Verification items for the finished model (mm, model axes). Face numbers are marked on the shaded views. A direction names the side the tool comes from. Coordinates: 2 decimals unless noted, no trailing zeros. Order: outer loops, then holes, each group sorted by start corner. A loop starts at its lowest first (then second) coordinate and runs counter-clockwise, first axis right, second up. Notation, with made-up numbers: M 57.25,-24 L 107.25,-24 A20 ccw 107.25,-15 Z; hole C -11.5,4 d9. An arc over 180 degrees is marked long. Write item = value, one per line.
```python
from build123d import *

# Parameters (mm, degrees)
BASE_FLANGE1_DEPTH = 2
EDGE_FLANGE1_DEPTH = 1017


# Sheet-metal steps are written as plain solids
with BuildPart() as part:
    # Sketch1 → Base-Flange1 (new body)
    with BuildSketch(Plane.XY):
        Polygon((960.416808149, 91.455857385), (985.416808149, 91.455857385), (985.416808149, 141.455857385), (-231.583191851, 141.455857385), (-231.583191851, 91.455857385), (-206.583191851, 91.455857385), (-206.583191851, -158.544142615), (960.416808149, -158.544142615), align=None)
    extrude(amount=-BASE_FLANGE1_DEPTH)

    # Edge-Flange1 section (across the edge) → Edge-Flange1 (add)
    with BuildSketch(Plane(origin=(-131.583191851, 142.192457385, -2), x_dir=(0, -1, 0), z_dir=(1, 0, 0))):
        with BuildLine():
            Line((-2, 0.7366), (-2, 13))
            Line((-2, 13), (0, 13))
            Line((0, 13), (0, 0.7366))
            ThreePointArc((0, 0.7366), (0.215745145, 0.215745145), (0.7366, 0))
            Line((0.7366, 0), (0.7366, -2))
            ThreePointArc((0.7366, -2), (-1.198468417, -1.198468417), (-2, 0.7366))
        make_face()
    extrude(amount=EDGE_FLANGE1_DEPTH)


solid = part.part
```
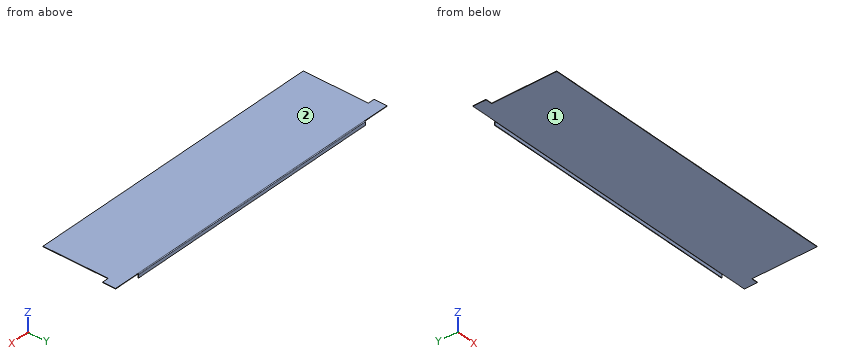
Item 1: Tool access check on the marked faces 1 and 2. Record the directions out of +Z, -Z, +X, -X, +Y, -Y that give a thin tool (end or side, any length) a straight path to the whole face; none if there is none.
Report:
face_1 = -Z, +X, -X, -Y
face_2 = +Z, +X, -X, +Y, -Y
Item 2: Gauge pin test, flat ends, axial feed: pin 1 (0.6 mm diameter, centred on y = -64, z = -1.5, fed in from +X); pin 2 (0.6 mm diameter, centred on x = -217, z = -1.5, fed in from -Y); pin 3 (1 mm diameter, centred on x = 959.5, z = -1, fed in from +Y); pin 4 (1 mm diameter, centred on x = 28, y = 19.5, fed in from +Z). Record the tip position at first contact, or that the pin passes through.
Report:
pin_1 = 960.42
pin_2 = 91.46
pin_3 = 141.46
pin_4 = 0
Item 3: Sectioned sample at B-B, the plane y = -36. Enter the section's corners in (x, z), then the cut area to 3 significant figures.
Report:
outline = M -206.58,-2 L 960.42,-2 L 960.42,0 L -206.58,0 Z
area = 2,330 mm^2
Item 4: Sectioned sample at A-A, the plane x = 249.5. Enter the section's corners in (y, z).
Report:
outline = M -158.54,-2 L 141.46,-2 A0.74 cw 142.19,-2.74 L 142.19,-15 L 144.19,-15 L 144.19,-2.74 A2.74 ccw 141.46,0 L -158.54,0 Z
Item 5: Sectioned sample at C-C, the plane z = -6.5. Enter the section's corners in (x, y).
Report:
outline = M -131.58,142.19 L 885.42,142.19 L 885.42,144.19 L -131.58,144.19 Z
Item 6: Scan lines: L1, parallel to Z at x = 896, y = -120.5; L2, parallel to Y at x = 102, z = -13; L3, parallel to X at y = 76, z = -1.75. Record each from-to range of solid material in increasing order. Write a range as from..to.
Report:
L1 = -2..0
L2 = 142.19..144.19
L3 = -206.58..960.42
